Geometry: final body of the model. Coordinates: model frame, mm. Face numbers are marked on the shaded views. A direction names the side the tool comes from. Give positions to 0.01 mm unless a question says otherwise; leave off trailing zeros. Write each loop counter-clockwise with the first axis right and the second up, starting at its lowest first coordinate (ties: lowest second). Pieces come first, ordered by that corner, then holes.
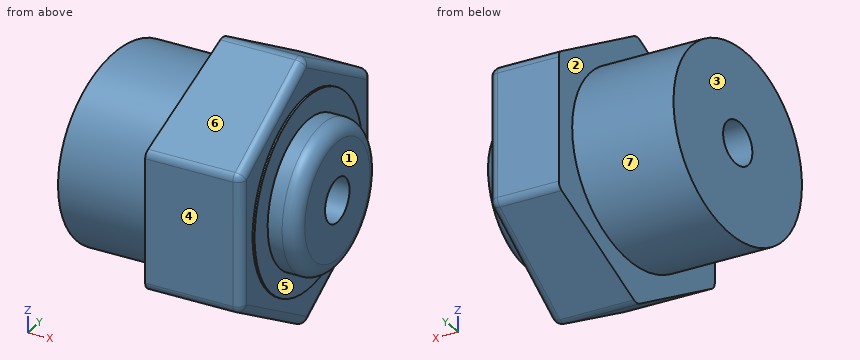
```python
from build123d import *

# Parameters (mm, degrees)
SALIENTE_EXTRUIR1_DEPTH = 3.33
REDONDEO1_R             = 0.3
CORTAR_EXTRUIR3_DEPTH   = 9.95
CROQUIS2_R              = 3.3
SALIENTE_EXTRUIR4_DEPTH = 3.4
CROQUIS6_R              = 2.5
SALIENTE_EXTRUIR5_DEPTH = 7.8
REDONDEO3_R             = 0.5
CROQUIS7_R              = 0.75
CORTAR_EXTRUIR4_DEPTH   = 10.871432541
CORTAR_EXTRUIR5_DEPTH   = 3.9


with BuildPart() as part:
    # Croquis1 → Saliente-Extruir1 (new body)
    with BuildSketch(Plane(origin=(0, 0, 0), x_dir=(0, 0, -1), z_dir=(1, 0, 0))):
        Polygon((-4.6, 0), (-2.3, -3.983716857), (2.3, -3.983716857), (4.6, 0), (2.3, 3.983716857), (-2.3, 3.983716857), align=None)
    extrude(amount=SALIENTE_EXTRUIR1_DEPTH)

    # Redondeo1
    redondeo1_edges = [part.edges().sort_by_distance(p)[0] for p in [
        (1.665, 3.983716857, 2.3),
        (1.665, 3.983716857, -2.3),
        (1.665, 0, -4.6),
        (1.665, -3.983716857, -2.3),
        (1.665, -3.983716857, 2.3),
        (1.665, 0, 4.6),
        (3.33, -3.983716857, 0),
        (3.33, -1.991858429, -3.45),
        (3.33, 1.991858429, -3.45),
        (3.33, 3.983716857, 0),
        (3.33, 1.991858429, 3.45),
        (3.33, -1.991858429, 3.45),
    ]]
    fillet(redondeo1_edges, radius=REDONDEO1_R)

    # Croquis5 → Cortar-Extruir3 (cut, symmetric)
    with BuildSketch(Plane.XY):
        Polygon((0, -3.983716857), (-2.185194876, -3.983716857), (-2.185194876, 4.171179011), (0.929133021, 4.171179011), align=None)
    extrude(amount=CORTAR_EXTRUIR3_DEPTH, both=True, mode=Mode.SUBTRACT)

    # Croquis2 → Saliente-Extruir4 (add, symmetric)
    with BuildSketch(Plane.ZY):
        with Locations(Location((0, 0, 0), (0, 0, 90))):
            Circle(CROQUIS2_R)
    extrude(amount=SALIENTE_EXTRUIR4_DEPTH, both=True)

    # Croquis6 → Saliente-Extruir5 (add)
    with BuildSketch(Plane.ZY.offset(3.4)):
        Circle(CROQUIS6_R)
    extrude(amount=-SALIENTE_EXTRUIR5_DEPTH)

    # Redondeo3
    redondeo3_edges = [part.edges().sort_by_distance(p)[0] for p in [
        (4.4, 0, -2.5),
    ]]
    fillet(redondeo3_edges, radius=REDONDEO3_R)

    # Croquis7 → Cortar-Extruir4 (cut, through all)
    with BuildSketch(Plane(origin=(4.4, 0, 0), x_dir=(0, 0, -1), z_dir=(1, 0, 0))):
        Circle(CROQUIS7_R)
    extrude(amount=-CORTAR_EXTRUIR4_DEPTH, mode=Mode.SUBTRACT)

    # Croquis8 → Cortar-Extruir5 (cut, symmetric)
    with BuildSketch(Plane.XY):
        Polygon((-3.4, -3.3), (-2.582609663, 4.139540535), (-3.4, 4.139540535), align=None)
    extrude(amount=CORTAR_EXTRUIR5_DEPTH, both=True, mode=Mode.SUBTRACT)


solid = part.part
```
Item 1: Pin query (flat end, axial travel): pin 1 Ø2 at (x, z) = (-0.5, -1) entering from +Y; pin 2 Ø1.7 at (y, z) = (0, 0) entering from -X; pin 3 Ø1 at (y, z) = (-1, -3) entering from -X; pin 4 Ø4 at (y, z) = (0, -3) entering from +X. Return the tip coordinate at first contact, or that it passes through.
Found:
pin 1: stops at y = 3.3
pin 2: stops at x = -3.13
pin 3: stops at x = -3.2
pin 4: stops at x = 4.4
Item 2: Line query: L1, parallel to Z at x = 1.25, y = 0; L2, parallel to Z at x = -0.75, y = 0; L3, parallel to Y at x = 2.75, z = 0. Output: solid intervals per line, ascending.
Found:
L1: z = -4.55 to -0.75, 0.75 to 4.55
L2: z = -3.3 to -0.75, 0.75 to 3.3
L3: y = -3.98 to -0.75, 0.75 to 3.98
Item 3: Reachability of the marked faces 5, 6 and 7 from +Z, -Z, +X, -X, +Y, -Y: full face, straight path, thin tool, end or side. Return the list, or none.
Found:
face 5: +X
face 6: +Z, +X, -X, -Y
face 7: -X
Item 4: Pull-direction query (Y, two-part tool) for the marked faces 1, 2, 3 and 4; classes: +Y half, -Y half, draft (parallel to the pull), parting line (faces both ways), or undercut.
Found:
face 1: draft
face 2: undercut
face 3: +Y half
face 4: -Y half
Item 5: Section A-A, the plane x = 2.5. Return the cut outline in (y, z), plus the area to 3 significant figures.
Found:
outline: (-3.98, -2.13) arc R0.3 ccw to (-3.83, -2.39) - (-0.15, -4.51) arc R0.3 ccw to (0.15, -4.51) - (3.83, -2.39) arc R0.3 ccw to (3.98, -2.13) - (3.98, 2.13) arc R0.3 ccw to (3.83, 2.39) - (0.15, 4.51) arc R0.3 ccw to (-0.15, 4.51) - (-3.83, 2.39) arc R0.3 ccw to (-3.98, 2.13) - close; hole circle Ø1.5 at (0, 0)
area: 53.2 mm2
Item 6: Section B-B, the plane x = -1.5. Return the cut outline in (y, z), plus the area to 3 significant figures.
Found:
outline: circle Ø6.6 at (0, 0); hole circle Ø1.5 at (0, 0)
area: 32.4 mm2
